Design review of the part shown in the three views and the two pictorial views. Dimensions are in mm from the part's minimum x, y and z. Give positions to 0.01 mm unless a question says otherwise; leave off trailing zeros. Order: outer loops, then holes, each group sorted by start corner. A loop starts at its lowest first (then second) coordinate and runs counter-clockwise, first axis right, second up.
Item 1: Consider section A-A (x = 128). Give the boundary of the cut face in (y, z).
Item 2: Consider section B-B (z = 38.5). Give the boundary of the cut face in (x, y).
Item 3: Consider section C-C (y = 2.25). Give the boundary of the cut face in (x, z), plus the area to 3 significant figures.
Item 4: For probe 1 along X at (y, z) = (1.15, 38.5) (1 decimal); probe 2 along X at (y, z) = (0.9, 40) (1 decimal); probe 3 along X at (y, z) = (2.75, 52) (1 decimal), list the stretches that pass through material, from the lowest coordinate up.
Item 5: Consider section D-D (x = 33.5). Give the boundary of the cut face in (y, z).
Item 6: For P1, Ø4, axis at x = 88, z = 38.5, coming from the -Y side (3 decimals), flat-tipped, find the tip position at first contact; note if it passes through.
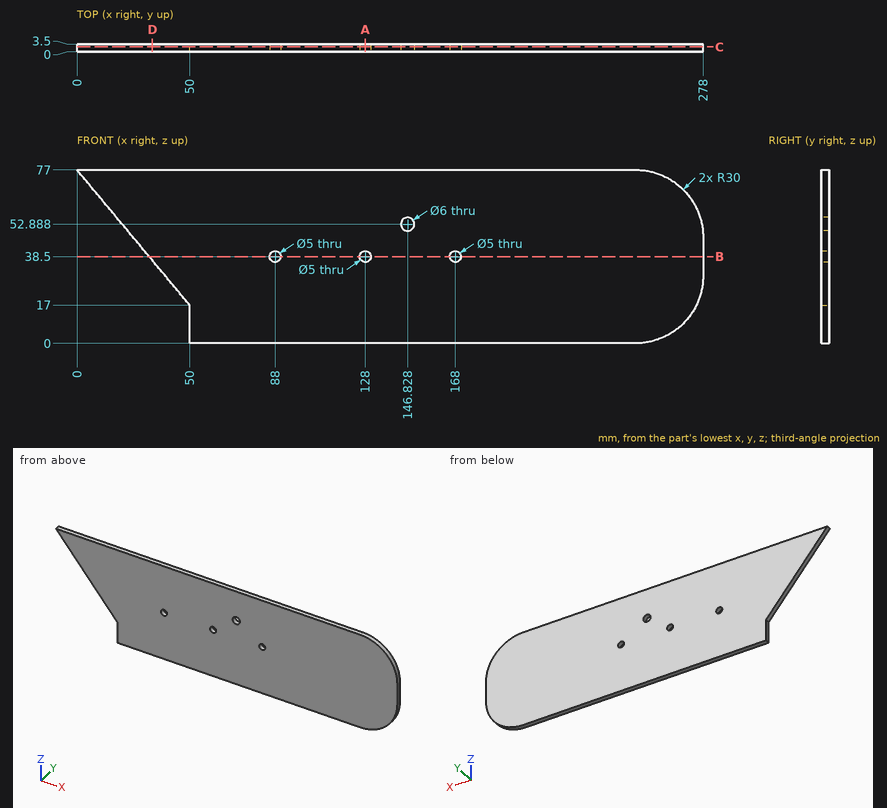
Resolved:
1. outline: (0, 0) - (3.5, 0) - (3.5, 36) - (0, 36) - close; (0, 41) - (3.5, 41) - (3.5, 77) - (0, 77) - close
2. outline: (32.08, 0) - (85.5, 0) - (85.5, 3.5) - (32.08, 3.5) - close; (90.5, 0) - (125.5, 0) - (125.5, 3.5) - (90.5, 3.5) - close; (130.5, 0) - (165.5, 0) - (165.5, 3.5) - (130.5, 3.5) - close; (170.5, 0) - (278, 0) - (278, 3.5) - (170.5, 3.5) - close
3. outline: (0, 77) - (50, 17) - (50, 0) - (248, 0) arc R30 ccw to (278, 30) - (278, 47) arc R30 ccw to (248, 77) - close; hole circle Ø5 at (88, 38.5); hole circle Ø5 at (128, 38.5); hole circle Ø6 at (146.83, 52.89); hole circle Ø5 at (168, 38.5)
3. area: 18,600 mm2
4. probe 1: x = 32.1 to 85.5, 90.5 to 125.5, 130.5 to 165.5, 170.5 to 278
4. probe 2: x = 30.8 to 86, 90 to 126, 130 to 166, 170 to 278
4. probe 3: x = 20.8 to 144, 149.7 to 277.6
5. outline: (0, 36.8) - (3.5, 36.8) - (3.5, 77) - (0, 77) - close
6. P1: passes through
